from build123d import *

# Parameters (mm, degrees)
SKETCH1_W           = 23
SKETCH1_H           = 17
BOSS_EXTRUDE1_DEPTH = 25
SKETCH2_W           = 21
SKETCH2_H           = 8
SKETCH2_W_2         = 3.15
SKETCH2_H_2         = 6
SKETCH2_W_3         = 3.3
SKETCH2_H_3         = 7.5
SKETCH2_W_4         = 4.3
SKETCH2_H_4         = 6.5
CUT_EXTRUDE1_DEPTH  = 29.801041648
CUT_EXTRUDE2_DEPTH  = 29.801041648
CUT_EXTRUDE3_REACH  = 30.953
SKETCH4_R           = 1.25


with BuildPart() as part:
    # Sketch1 → Boss-Extrude1 (new body)
    with BuildSketch(Plane(origin=(0, 0, 0), x_dir=(1, 0, 0), z_dir=(0, 1, 0))):
        Rectangle(SKETCH1_W, SKETCH1_H)
    extrude(amount=BOSS_EXTRUDE1_DEPTH)

    # Sketch2 → Cut-Extrude1 (cut, through all)
    with BuildSketch(Plane(origin=(0, 25, 0), x_dir=(1, 0, 0), z_dir=(0, 1, 0))):
        with Locations((0, -4.5)):
            Rectangle(SKETCH2_W, SKETCH2_H)
        with Locations((-8.925, 5.5)):
            Rectangle(SKETCH2_W_2, SKETCH2_H_2)
        with Locations((-4.75, 4.75)):
            Rectangle(SKETCH2_W_3, SKETCH2_H_3)
        with Locations((0, 5.25)):
            Rectangle(SKETCH2_W_4, SKETCH2_H_4)
        with Locations((4.75, 4.75)):
            Rectangle(SKETCH2_W_3, SKETCH2_H_3)
        with Locations((8.925, 5.5)):
            Rectangle(SKETCH2_W_2, SKETCH2_H_2)
    extrude(amount=-CUT_EXTRUDE1_DEPTH, mode=Mode.SUBTRACT)

    # Sketch3 → Cut-Extrude2 (cut, through all)
    with BuildSketch(Plane(origin=(0, 25, 0), x_dir=(1, 0, 0), z_dir=(0, 1, 0))):
        with BuildLine():
            Line((8.35, 2.5), (8.35, 1.65))
            ThreePointArc((8.35, 1.65), (9, 1), (9.65, 1.65))
            Line((9.65, 1.65), (9.65, 2.5))
            Line((9.65, 2.5), (8.35, 2.5))
        make_face()
        with BuildLine():
            Line((-8.35, 2.5), (-8.35, 1.65))
            ThreePointArc((-8.35, 1.65), (-9, 1), (-9.65, 1.65))
            Line((-9.65, 1.65), (-9.65, 2.5))
            Line((-9.65, 2.5), (-8.35, 2.5))
        make_face()
    extrude(amount=-CUT_EXTRUDE2_DEPTH, mode=Mode.SUBTRACT)

    # Sketch4 → Cut-Extrude3 (cut, up to next)
    with BuildSketch(Plane.XY.offset(0.5), mode=Mode.PRIVATE) as cut_extrude3_sk1:
        with Locations((0, 19)):
            Circle(SKETCH4_R)
    cut_extrude3_tool1 = extrude(cut_extrude3_sk1.sketch, amount=-CUT_EXTRUDE3_REACH, mode=Mode.PRIVATE) & part.part
    add(cut_extrude3_tool1.solids().sort_by_distance((0, 19, 0.5))[0], mode=Mode.SUBTRACT)


solid = part.part
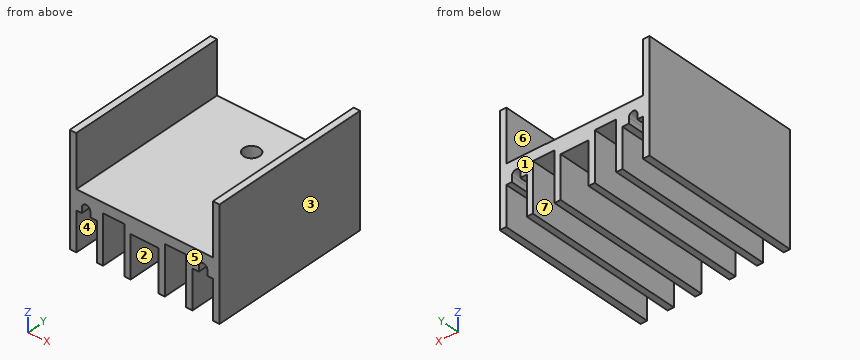
For this review, take the finished solid that the model builds, in its own axes (mm). Face numbers are marked on the shaded views. A direction names the side the tool comes from. Coordinates: 2 decimals unless noted, no trailing zeros. Loops run counter-clockwise (first coordinate to the right, second up) from the corner with the lowest first, then second, coordinate; pieces in that order, holes last. Notation, with made-up numbers: (15, -22.75) - (55, -22.75) arc R17 ccw to (55, -5.75) - close; hole circle Ø5 at (-24, -4). An arc over 180 degrees is marked (long way). Return JSON: item names as keys, results as strings.
Item 1: For line 1 (X direction, y = 21.25, z = -3.5); line 2 (Y direction, x = 0, z = -0.7); line 3 (X direction, y = 21.5, z = 5), list the stretches that pass through material, from the lowest coordinate up.
Determined:
{"line 1": "x = -11.5 to -10.5, -7.35 to -6.4, -3.1 to -2.15, 2.15 to 3.1, 6.4 to 7.35, 10.5 to 11.5", "line 2": "y = 0 to 17.75, 20.25 to 25", "line 3": "x = -11.5 to -10.5, 10.5 to 11.5"}
Item 2: Insertion check: pin 1 (2 mm diameter, centred on x = 7.5, y = 11.5, fed in from +Z); pin 2 (1 mm diameter, centred on x = 1.5, y = 16.5, fed in from -Z); pin 3 (1 mm diameter, centred on x = -5, y = 14, fed in from -Z); pin 4 (1.5 mm diameter, centred on x = 9, z = 4.5, fed in from -Y). Each pin has a flat end and moves straight along its axis. Give the tip position at first contact, or say it passes through.
Determined:
{"pin 1": "stops at z = 0.5", "pin 2": "stops at z = -2", "pin 3": "stops at z = -1", "pin 4": "passes through"}
Item 3: Take a section at D-D (x = -2.75). Give the boundary of the cut face in (y, z).
Determined:
{"outline": "(0, -8.5) - (25, -8.5) - (25, 0.5) - (0, 0.5) - close"}
Item 4: Take a section at B-B (z = 5). Give the boundary of the cut face in (x, y), then the cut area to 3 significant figures.
Determined:
{"outline": "(-11.5, 0) - (-10.5, 0) - (-10.5, 25) - (-11.5, 25) - close; (10.5, 0) - (11.5, 0) - (11.5, 25) - (10.5, 25) - close", "area": "50.0 mm2"}
Item 5: Take a section at A-A (x = 0). Give the boundary of the cut face in (y, z), then the cut area to 4 significant figures.
Determined:
{"outline": "(0, -2) - (17.75, -2) - (17.75, 0.5) - (0, 0.5) - close; (20.25, -2) - (25, -2) - (25, 0.5) - (20.25, 0.5) - close", "area": "56.25 mm2"}
Item 6: For the marked faces 5, 6 and 7, list the 3-axis set-ups (+Z, -Z, +X, -X, +Y, -Y) from which the entire face can be reached by the end or side of a thin tool; tool diameter is ignored.
Determined:
{"face 5": "+Z, -Z, +X, -X, -Y", "face 6": "+Z, +Y, -Y", "face 7": "-Z, +Y, -Y"}
Item 7: Take a section at C-C (z = -6.75). Give the boundary of the cut face in (x, y).
Determined:
{"outline": "(-11.5, 0) - (-10.5, 0) - (-10.5, 25) - (-11.5, 25) - close; (-7.35, 0) - (-6.4, 0) - (-6.4, 25) - (-7.35, 25) - close; (-3.1, 0) - (-2.15, 0) - (-2.15, 25) - (-3.1, 25) - close; (2.15, 0) - (3.1, 0) - (3.1, 25) - (2.15, 25) - close; (6.4, 0) - (7.35, 0) - (7.35, 25) - (6.4, 25) - close; (10.5, 0) - (11.5, 0) - (11.5, 25) - (10.5, 25) - close"}
Item 8: Mouldability with a two-part tool opening along X and no side actions: class the marked faces 1, 2, 3 and 4 as pulls with the +X half, pulls with the -X half, needs draft (parallel to the pull), parting line crosses it, or undercut.
Determined:
{"face 1": "needs draft", "face 2": "undercut", "face 3": "pulls with the +X half", "face 4": "undercut"}
